Autodesk Fusion 360 part; units mm, degrees
sketch "Sketch1" plane through (0, 0, 0) normal (1, 0, 0) x (0, 1, 0)
  circle A0 centre (0, 0) radius 3.58
  circle A1 centre (16, 0) radius 2
  line L0 (0.3535, 3.5625) -> (16.1975, 1.9902)
  line L1 (0.3535, -3.5625) -> (16.1975, -1.9902)
  circle A2 centre (16, 0) radius 0.5
  circle A3 centre (14, 0) radius 0.5
  circle A4 centre (12, 0) radius 0.5
  circle A5 centre (10, 0) radius 0.5
  circle A6 centre (8, 0) radius 0.5
  line L2 (0, 7) -> (0, -7.5)
  circle A7 centre (-8, 0) radius 0.5
  circle A8 centre (-10, 0) radius 0.5
  line L3 (-0.3535, 3.5625) -> (-16.1975, 1.9902)
  circle A9 centre (-12, 0) radius 0.5
  circle A10 centre (-14, 0) radius 0.5
  circle A11 centre (-16, 0) radius 2
  circle A12 centre (-16, 0) radius 0.5
  line L4 (-0.3535, -3.5625) -> (-16.1975, -1.9902)
  dimension "d4" = 7.16
  dimension "d5" = 4
  dimension "d6" = 16
  dimension "d7" = 1
  dimension "d10" = -8
  dimension "d11" = 0
extrude "Extrude1" add sketch "Sketch1" along normal blind 1.8 contours A0 L2 | A0 A1 L0 L1 A3 | A0 L2 | A1 A3 | A0 L3 A10 A11 L4 | A10 A11 picked at (14.8153, -0.6023) picked at (-14.8153, -0.6023) makes body 1
extrude "Extrude2" add sketch "Sketch1" along normal blind 1.8 separate body contours A0 L2 | A0 A1 L0 L1 A3 | A0 L2 | A1 A3 picked at (14.8153, -0.6023) makes body 2
sketch "Sketch2" plane through (0, 0, 0) normal (1, 0, 0) x (0, 1, 0)
extrude "Extrude3" add sketch "Sketch1" against normal blind 1.83 contours A0 L2 | A0 L2 bodies 1
sketch "Sketch3" plane through (1.8, 0, 0) normal (1, 0, 0) x (0, 1, 0)
  circle A0 centre (-10, 0) radius 0.5
  circle A1 centre (10, 0) radius 0.5
  circle A2 centre (-12, 0) radius 0.5
  circle A3 centre (12, 0) radius 0.5
  circle A4 centre (-8, 0) radius 0.5
  circle A5 centre (16, 0) radius 0.5
  circle A6 centre (-16, 0) radius 0.5
  circle A7 centre (14, 0) radius 0.5
  circle A8 centre (8, 0) radius 0.5
  circle A9 centre (-14, 0) radius 0.5
  line L0 (0.3535, -3.5625) -> (16.1975, -1.9902)
  arc A10 (16.1975, -1.9902) -> (16.1975, 1.9902) centre (16, 0) ccw
  line L1 (16.1975, 1.9902) -> (0.3535, 3.5625)
  arc A11 (0.3535, 3.5625) -> (-0.3535, 3.5625) centre (0, 0) ccw
  line L2 (-0.3535, 3.5625) -> (-16.1975, 1.9902)
  arc A12 (-16.1975, 1.9902) -> (-16.1975, -1.9902) centre (-16, 0) ccw
  line L3 (-16.1975, -1.9902) -> (-0.3535, -3.5625)
  arc A13 (-0.3535, -3.5625) -> (0.3535, -3.5625) centre (0, 0) ccw
  circle A14 centre (0, 0) radius 2.5
  circle A15 centre (0, 0) radius 3.58
  dimension "d18" = 5
extrude "Extrude4" cut sketch "Sketch3" against normal blind 0.8 contours A14 bodies 1
sketch "Sketch4" plane through (1, 0, 0) normal (1, 0, 0) x (0, 1, 0)
  circle A0 centre (0, 0) radius 2.5
  circle A1 centre (0, 0) radius 2.5
  circle A2 centre (0, 0) radius 1
  dimension "d21" = 2
extrude "Extrude5" cut sketch "Sketch4" against normal blind 13.5 contours A2 bodies 1
sketch "Sketch5" plane through (-1.83, 0, 0) normal (-1, 0, 0) x (0, -1, 0)
  circle A0 centre (0, 0) radius 1
  circle A1 centre (0, 0) radius 3.58
  circle A2 centre (0, 0) radius 2.3
  dimension "d24" = 4.6
extrude "Extrude6" cut sketch "Sketch5" against normal blind 1.5 contours A2 bodies 1
extrude "Extrude7" add sketch "Sketch1" against normal blind 1.83 contours A0 L2 | A0 L2 bodies 2
extrude "Extrude8" cut sketch "Sketch3" against normal blind 0.8 contours A14 bodies 2
extrude "Extrude9" cut sketch "Sketch5" against normal blind 1.5 contours A2 bodies 2
extrude "Extrude10" cut 1 faces at (-1.83, 0.6188, -0.2429) along direction (1, 0, 0) blind 27.5 on bodies 2 bodies 2
hidden bodies 1
equation "d4 = 3.58 * 2 mm"
equation "d16 = -3.43 mm + 1.6 mm"
equation "d27 = -3.43 mm + 1.6 mm"
Geometry: final body of the model. Coordinates: model frame, mm. A direction names the side the tool comes from. Give positions to 0.01 mm unless a question says otherwise; leave off trailing zeros. Write each loop counter-clockwise with the first axis right and the second up, starting at its lowest first coordinate (ties: lowest second). Pieces come first, ordered by that corner, then holes.
1. Section query D-D, the plane y = 2.75. Return loops of the section in (x, z), then the cut area to 3 significant figures.
2. Reachability of faces 1 (the cylindrical face through (-1.09, 1.825, -1.4)), 2 (the cylindrical face through (0.9, 9.5, 0)), 3 (the flat face through (1, 1, -1)) from +Z, -Z, +X, -X, +Y, -Y: full face, straight path, thin tool, end or side. Return the list, or none.
3. Pin query (flat end, axial travel): P1, Ø2, axis at y = 12, z = -0.5, coming from the -X side; P2, Ø2.5, axis at y = 1, z = 0, coming from the +X side; P3, Ø1.5, axis at x = -1, z = 1.5, coming from the +Y side. Return the tip coordinate at first contact, or that it passes through.
4. Line query: probe 1 along Z at (x, y) = (0.1, 0); probe 2 along X at (y, z) = (1, -0.5); probe 3 along Z at (x, y) = (0.4, 10). Output: solid intervals per line, ascending.
5. Section query C-C, the plane z = 0. Count the separate pieces of the cut face and the enclosed holes in it, then the cut area to 3 significant figures.
6. Draft query along Y for faces 4 (the flat face through (0.887, 8.165, -2.787)), 5 (the cylindrical face through (0.9, 11.5, 0)), 6 (the flat face through (-1.83, 2.34, -0.75)). Return one class per face: released by +Y, released by -Y, zero draft, split by the parting line, or undercut.
7. Section query A-A, the plane x = 0.3. Return loops of the section in (y, z).
8. Section query B-B, the plane y = 8. Return loops of the section in (x, z), then the cut area to 3 significant figures.
Computed:
1. outline: (-1.83, -2.29) - (0, -2.29) - (0, -3.32) - (1.8, -3.32) - (1.8, 3.32) - (0, 3.32) - (0, 2.29) - (-1.83, 2.29) - close
1. area: 20.4 mm2
2. face 1: -X
2. face 2: +X, -X
2. face 3: +X
3. P1: stops at x = 0
3. P2: stops at x = 1
3. P3: stops at y = 3.5
4. probe 1: z = -3.58 to -1, 1 to 3.58
4. probe 2: x = -0.33 to 1
4. probe 3: z = -2.61 to -0.5, 0.5 to 2.61
5. separate pieces: 7
5. enclosed holes: 0
5. area: 29.4 mm2
6. face 4: released by +Y
6. face 5: undercut
6. face 6: zero draft
7. outline: (0.35, -3.56) - (16.2, -1.99) arc R2 ccw to (16.2, 1.99) - (0.35, 3.56) arc R3.58 ccw (long way) to start; hole circle Ø2 at (0, 0); hole circle Ø1 at (8, 0); hole circle Ø1 at (10, 0); hole circle Ø1 at (12, 0); hole circle Ø1 at (14, 0); hole circle Ø1 at (16, 0)
8. outline: (0, -2.8) - (1.8, -2.8) - (1.8, -0.5) - (0, -0.5) - close; (0, 0.5) - (1.8, 0.5) - (1.8, 2.8) - (0, 2.8) - close
8. area: 8.29 mm2
